```python
from build123d import *

# Parameters (mm, degrees)
F0_W      = 55
F0_H      = 55
F1_DEPTH  = 55
F2_SIZE   = 5
F5_T      = -2.5
F7_DEPTH  = 2.5
F4_R      = 5
F8_DEPTH  = 2.5
F3_R      = 5
F9_DEPTH  = 2.5
F10_R     = 7.5
F11_DEPTH = 7


with BuildPart() as f1:
    # F0 (on Front) → F1 (new body)
    with BuildSketch(Plane.XZ):
        Rectangle(F0_W, F0_H)
    extrude(amount=F1_DEPTH)

    # F2
    f2_edges = [f1.edges().sort_by_distance(p)[0] for p in [
        (27.5, -27.5, 27.5),
        (-27.5, -27.5, 27.5),
        (27.5, -27.5, -27.5),
        (-27.5, -27.5, -27.5),
    ]]
    chamfer(f2_edges, length=F2_SIZE)

    # F5
    f5_openings = [f1.faces().sort_by_distance(p)[0] for p in [
        (0, -55, 0),
    ]]
    offset(amount=F5_T, openings=f5_openings)

    # F6 (on face) → F7 (join)
    with BuildSketch(Plane.XZ.offset(55)):
        Polygon((27.5, 22.5), (22.5, 27.5), (-22.5, 27.5), (-27.5, 22.5), (-27.5, -22.5), (-22.5, -27.5), (22.5, -27.5), (27.5, -22.5), align=None)
    extrude(amount=-F7_DEPTH)

    # F4 (on face) → F8 (cut)
    with BuildSketch(Plane.YZ.offset(27.5)):
        with Locations((-27.5, 0)):
            Circle(F4_R)
    extrude(amount=-F8_DEPTH, mode=Mode.SUBTRACT)

    # F3 (on face) → F9 (cut)
    with BuildSketch(Plane.XZ.offset(55)):
        Circle(F3_R)
    extrude(amount=-F9_DEPTH, mode=Mode.SUBTRACT)

    # F10 (on face) → F11 (join)
    with BuildSketch(Plane(origin=(0, 0, 0), x_dir=(-1, 0, 0), z_dir=(0, 1, 0))):
        Circle(F10_R)
    extrude(amount=F11_DEPTH)


solid = f1.part
```
Design review of the part built by this model. Coordinates are the model's own, in mm. A direction names the side the tool comes from. Round coordinates to 2 decimals unless told otherwise and drop trailing zeros. Write each loop counter-clockwise with the first axis right and the second up, starting at its lowest first coordinate (ties: lowest second). Pieces come first, ordered by that corner, then holes.
Item 1: We need section B-B on y = -50. Write out the cut boundary in (x, z), and give its area (3 significant figures).
Item 2: We need section D-D on x = -18. Write out the cut boundary in (y, z).
Item 3: For faces 1 (the flat face through (-6, 0, 6)), 2 (the flat face through (23.257, -27.15, -23.207)), 3 (the cylindrical face through (-1.08, -53.77, -4.88)), list the 3-axis set-ups (+Z, -Z, +X, -X, +Y, -Y) from which the entire face can be reached by the end or side of a thin tool; tool diameter is ignored.
Item 4: Clearance check with flat-ended pins moving along their axes: pin 1 Ø3 at (x, z) = (0, 4) entering from -Y; pin 2 Ø6 at (x, z) = (0, 0) entering from -Y; pin 3 Ø4 at (x, z) = (-9.5, -4.5) entering from +Y. State where each tip first meets the part, or that it passes through.
Item 5: We need section C-C on z = -15.5. Write out the cut boundary in (x, y).
Item 6: The part is to be moulded in two halves that separate along X. For faces 4 (the flat face through (-25, -27, -25)), 5 (the flat face through (25, -27, -25)), 6 (the flat face through (-23.207, -27.15, 23.257)), say which applies: +X half, -X half, draft (parallel to the pull), parting line (faces both ways), or undercut.
Item 7: We need section A-A on z = 0. Write out the cut boundary in (x, y).
Item 8: For probe 1 along X at (y, z) = (-3.5, -1.5); probe 2 along Y at (x, z) = (20.5, 6.5); probe 3 along Z at (x, y) = (0, -53.6), list the stretches that pass through material, from the lowest coordinate up.
Returned:
1. outline: (-27.5, -22.5) - (-22.5, -27.5) - (22.5, -27.5) - (27.5, -22.5) - (27.5, 22.5) - (22.5, 27.5) - (-22.5, 27.5) - (-27.5, 22.5) - close; hole (-25, -21.46) - (-21.46, -25) - (21.46, -25) - (25, -21.46) - (25, 21.46) - (21.46, 25) - (-21.46, 25) - (-25, 21.46) - close
1. area: 500 mm2
2. outline: (-55, -27.5) - (0, -27.5) - (0, 27.5) - (-55, 27.5) - close; hole (-52.5, -25) - (-2.5, -25) - (-2.5, 25) - (-52.5, 25) - close
3. face 1: +Y
3. face 2: none
3. face 3: -Y
4. pin 1: stops at y = -55
4. pin 2: stops at y = -2.5
4. pin 3: stops at y = 0
5. outline: (-27.5, -55) - (27.5, -55) - (27.5, 0) - (-27.5, 0) - close; hole (-25, -52.5) - (25, -52.5) - (25, -2.5) - (-25, -2.5) - close
6. face 4: -X half
6. face 5: +X half
6. face 6: undercut
7. outline: (-27.5, -55) - (-5, -55) - (-5, -52.5) - (-25, -52.5) - (-25, -2.5) - (25, -2.5) - (25, -22.5) - (27.5, -22.5) - (27.5, 0) - (7.5, 0) - (7.5, 7) - (-7.5, 7) - (-7.5, 0) - (-27.5, 0) - close; (5, -55) - (27.5, -55) - (27.5, -32.5) - (25, -32.5) - (25, -52.5) - (5, -52.5) - close
8. probe 1: x = -27.5 to -25, 25 to 27.5
8. probe 2: y = -55 to -52.5, -2.5 to 0
8. probe 3: z = -27.5 to -5, 5 to 27.5
